Could you check a few things on this drawing? It's one solid part, dimensions in mm from its lowest x, y, z. Coordinates: 2 decimals unless noted, no trailing zeros. Order: outer loops, then holes, each group sorted by start corner. A loop starts at its lowest first (then second) coordinate and runs counter-clockwise, first axis right, second up.
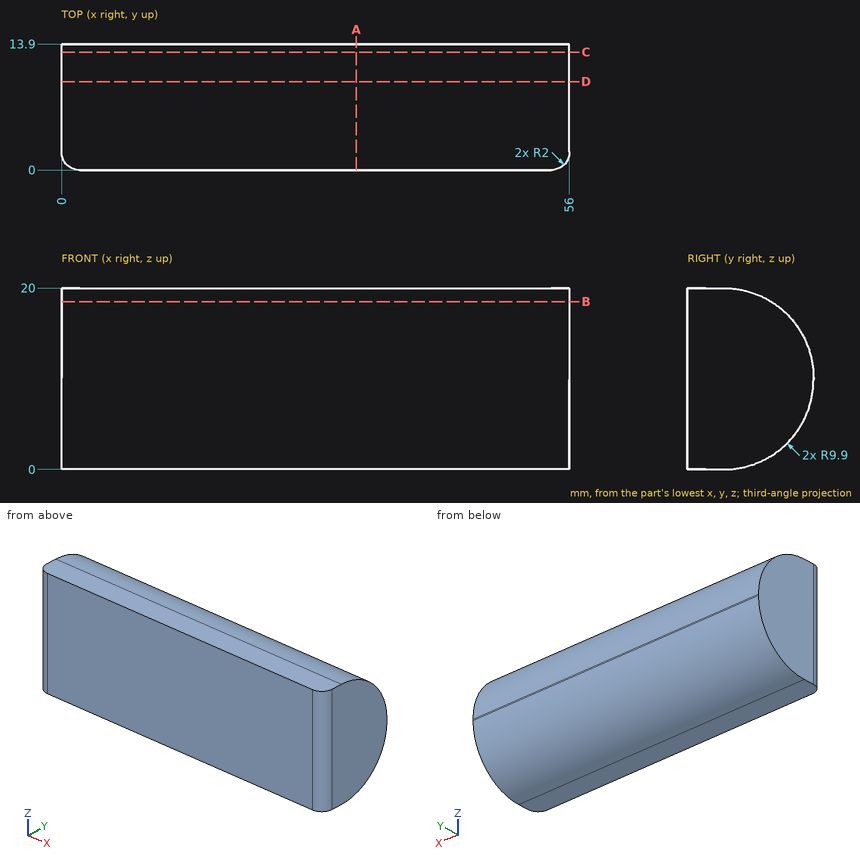
Item 1: For pin 1 Ø4 at (x, y) = (49, 8) entering from -Z; pin 2 Ø5 at (x, y) = (12.5, 12) entering from -Z; pin 3 Ø5 at (x, y) = (12, 9) entering from -Z, each with a flat end and sliding along its axis, tell me the tip position at first contact or that it passes through.
Item 2: Suppose I cut it at A-A (x = 32.5). List the corners of the cut face in (y, z) for me.
Item 3: I need wall thicknesses on line 1 (Z direction, x = 2.5, y = 12); line 2 (Y direction, x = 3, z = 16); line 3 (Y direction, x = 35.5, z = 3.5). Which ranges of each line are inside material? Lowest first, please.
Item 4: Suppose I cut it at D-D (y = 9.75). List the corners of the cut face in (x, z) for me.
Item 5: Suppose I cut it at C-C (y = 13). List the corners of the cut face in (x, z) for me.
Item 6: Suppose I cut it at B-B (z = 18.5). List the corners of the cut face in (x, y) for me.
Geometry results:
1. pin 1: stops at z = 0.2
1. pin 2: stops at z = 1.67
1. pin 3: stops at z = 0.32
2. outline: (0, 0) - (4, 0) arc R9.9 ccw to (13.9, 9.9) - (13.9, 10.1) arc R9.9 ccw to (4, 20) - (0, 20) - close
3. line 1: z = 4.07 to 15.93
3. line 2: y = 0 to 11.95
3. line 3: y = 0 to 11.55
4. outline: (0, 1.84) - (56, 1.84) - (56, 18.16) - (0, 18.16) - close
5. outline: (0, 5.78) - (56, 5.78) - (56, 14.22) - (0, 14.22) - close
6. outline: (0, 2) arc R2 ccw to (2, 0) - (54, 0) arc R2 ccw to (56, 2) - (56, 9.24) - (0, 9.24) - close
